```python
from build123d import *

# Parameters (mm, degrees)
SKETCH_1_R              = 2.1
F_20XS5_20X40S5_1_DEPTH = 690


with BuildPart() as part:
    # 草图1 → 20xs5 20X40S5(1) (new body)
    with BuildSketch(Plane.YZ):
        with BuildLine():
            Line((-10, 19), (-10, 13.3))
            ThreePointArc((-10, 13.3), (-9.912132034, 13.087867966), (-9.7, 13))
            Line((-9.7, 13), (-8, 13))
            Line((-8, 13), (-8, 16))
            Line((-8, 16), (-7.060660172, 16))
            Line((-7.060660172, 16), (-4, 12.939339828))
            Line((-4, 12.939339828), (-4, 7.060660172))
            Line((-4, 7.060660172), (-7.060660172, 4))
            Line((-7.060660172, 4), (-8, 4))
            Line((-8, 4), (-8, 7))
            Line((-8, 7), (-9.7, 7))
            ThreePointArc((-9.7, 7), (-9.912132034, 6.912132034), (-10, 6.7))
            Line((-10, 6.7), (-10, -6.7))
            ThreePointArc((-10, -6.7), (-9.912132034, -6.912132034), (-9.7, -7))
            Line((-9.7, -7), (-8, -7))
            Line((-8, -7), (-8, -4))
            Line((-8, -4), (-7.060660172, -4))
            Line((-7.060660172, -4), (-4, -7.060660172))
            Line((-4, -7.060660172), (-4, -12.939339828))
            Line((-4, -12.939339828), (-7.060660172, -16))
            Line((-7.060660172, -16), (-8, -16))
            Line((-8, -16), (-8, -13))
            Line((-8, -13), (-9.7, -13))
            ThreePointArc((-9.7, -13), (-9.912132034, -13.087867966), (-10, -13.3))
            Line((-10, -13.3), (-10, -19))
            ThreePointArc((-10, -19), (-9.948683298, -19.316227766), (-9.8, -19.6))
            Line((-9.8, -19.6), (-3, -19.6))
            Line((-3, -19.6), (-3, -18))
            Line((-3, -18), (-6, -18))
            Line((-6, -18), (-6, -17.060660172))
            Line((-6, -17.060660172), (-2.939339828, -14))
            Line((-2.939339828, -14), (2.939339828, -14))
            Line((2.939339828, -14), (6, -17.060660172))
            Line((6, -17.060660172), (6, -18))
            Line((6, -18), (3, -18))
            Line((3, -18), (3, -19.6))
            Line((3, -19.6), (9.8, -19.6))
            ThreePointArc((9.8, -19.6), (9.948683298, -19.316227766), (10, -19))
            Line((10, -19), (10, -13.3))
            ThreePointArc((10, -13.3), (9.912132034, -13.087867966), (9.7, -13))
            Line((9.7, -13), (8, -13))
            Line((8, -13), (8, -16))
            Line((8, -16), (7.060660172, -16))
            Line((7.060660172, -16), (4, -12.939339828))
            Line((4, -12.939339828), (4, -7.060660172))
            Line((4, -7.060660172), (7.060660172, -4))
            Line((7.060660172, -4), (8, -4))
            Line((8, -4), (8, -7))
            Line((8, -7), (9.7, -7))
            ThreePointArc((9.7, -7), (9.912132034, -6.912132034), (10, -6.7))
            Line((10, -6.7), (10, 6.7))
            ThreePointArc((10, 6.7), (9.912132034, 6.912132034), (9.7, 7))
            Line((9.7, 7), (8, 7))
            Line((8, 7), (8, 4))
            Line((8, 4), (7.060660172, 4))
            Line((7.060660172, 4), (4, 7.060660172))
            Line((4, 7.060660172), (4, 12.939339828))
            Line((4, 12.939339828), (7.060660172, 16))
            Line((7.060660172, 16), (8, 16))
            Line((8, 16), (8, 13))
            Line((8, 13), (9.7, 13))
            ThreePointArc((9.7, 13), (9.912132034, 13.087867966), (10, 13.3))
            Line((10, 13.3), (10, 19))
            ThreePointArc((10, 19), (9.948683298, 19.316227766), (9.8, 19.6))
            Line((9.8, 19.6), (3, 19.6))
            Line((3, 19.6), (3, 18))
            Line((3, 18), (6, 18))
            Line((6, 18), (6, 17.060660172))
            Line((6, 17.060660172), (2.939339828, 14))
            Line((2.939339828, 14), (-2.939339828, 14))
            Line((-2.939339828, 14), (-6, 17.060660172))
            Line((-6, 17.060660172), (-6, 18))
            Line((-6, 18), (-3, 18))
            Line((-3, 18), (-3, 19.6))
            Line((-3, 19.6), (-9.8, 19.6))
            ThreePointArc((-9.8, 19.6), (-9.948683298, 19.316227766), (-10, 19))
        make_face()
        with Locations((0, -10)):
            Circle(SKETCH_1_R, mode=Mode.SUBTRACT)
        with Locations((0, 10)):
            Circle(SKETCH_1_R, mode=Mode.SUBTRACT)
        Polygon((-8, -2.5), (-6.439339828, -2.5), (-2.939339828, -6), (2.939339828, -6), (6.439339828, -2.5), (8, -2.5), (8, 2.5), (6.439339828, 2.5), (2.939339828, 6), (-2.939339828, 6), (-6.439339828, 2.5), (-8, 2.5), align=None, mode=Mode.SUBTRACT)
    extrude(amount=F_20XS5_20X40S5_1_DEPTH)


solid = part.part
```
Input: part model. Units: mm. Frame: model coordinates. Round coordinates to 2 decimals unless told otherwise and drop trailing zeros. One line per item, written item: value. Start each with the question number.
(1) Contact query for a flat-ended pin moving along its axis: P1, Ø3, axis at x = 320, y = -1, coming from the +Z side. Output: stop coordinate, or through.
(2) Section A-A, the plane x = 315.5. Count the separate pieces of the cut face and the enclosed holes in it, plus the area to 3 significant figures.
(3) Ray query, line 1 (Z direction, x = 442.5, y = 0); line 2 (Y direction, x = 294, z = 1); line 3 (Z direction, x = 439.5, y = 5.5). Return the intervals inside material, ascending. Write a range as [from, to].
Results below:
1. P1: z = 14
2. separate pieces: 1
2. enclosed holes: 3
2. area: 311 mm^2
3. line 1: [-14, -12.1], [-7.9, -6], [6, 7.9], [12.1, 14]
3. line 2: [-10, -8], [8, 10]
3. line 3: [-19.6, -18], [-16.56, -14.44], [-5.56, -3.44], [3.44, 5.56], [14.44, 16.56], [18, 19.6]
